Can you work these out from the model? Positions are in its coordinate system, mm. A direction names the side the tool comes from. Round coordinates to 2 decimals unless told otherwise and drop trailing zeros. Order: outer loops, then holes, each group sorted by start corner. A loop starts at its lowest first (then second) coordinate and runs counter-clockwise, first axis right, second up.
Q1. If we section it at C-C (y = 42): Please give me the cut outline in (x, z), plus the area to 3 significant figures.
Q2. If we section it at D-D (z = 2.1): Please give me the cut outline in (x, y).
Q3. If we section it at A-A (x = 8): Please give me the cut outline in (y, z).
Q4. If we section it at B-B (y = 8): Please give me the cut outline in (x, z).
Q5. Will these pins go through, and if not, where does the flat tip stop? P1, Ø1, axis at x = 25, z = 2.5, coming from the +Y side; P2, Ø2.5, axis at x = 42, y = 42, coming from the +Z side.
Q6. We'd pull the mould along Y, two halves only. Please class faces 1 (the face through (14, 25, 1)), 2 (the face through (30, 20, 0)), 3 (the face through (42, 44, 2)), 4 (the face through (0.86, 0.9, 1.52)): pulls with the +Y half, pulls with the -Y half, needs draft (parallel to the pull), parting line crosses it, or undercut.
Q7. If I drill on line 1 (X direction, y = 42, z = 1); line 2 (Y direction, x = 42, z = 2.2); line 3 (Y direction, x = 8, z = 1.2), over which ranges is the centre line in solid material (lowest first)?
Q8. For faces 5 (the face through (46.99, 2.85, 1.52)), 6 (the face through (25, 37, 1)), which set-ups out of +Z, -Z, +X, -X, +Y, -Y let a thin tool reach every point of the face, with its end or its side?
Autodesk Fusion 360 part; units mm, degrees
sketch "Sketch1" plane through (0, 0, 0) normal (0, 0, 1) x (1, 0, 0)
  line L0 (0, 0) -> (50, 0)
  line L1 (50, 0) -> (50, 50)
  line L2 (50, 50) -> (25, 50)
  line L3 (25, 50) -> (25, 25)
  line L4 (25, 25) -> (0, 25)
  line L5 (0, 25) -> (0, 0)
  line L6 (-25, 0) -> (-25, 55) construction
  dimension "d1" = 25
  dimension "d2" = 25
  dimension "d3" = 50
  dimension "d4" = 50
extrude "Extrude1" add sketch "Sketch1" along normal blind 3
ref_plane "WorkPlane1" through (-30, 0, 0) normal (1, 0, 0) x (0, 1, 0)
sketch "Sketch2" plane through (0, 0, 3) normal (0, 0, 1) x (-1, 0, 0)
  line L0 (0, -25) -> (0, 0)
  line L1 (0, 0) -> (-50, 0)
  line L2 (-50, 0) -> (-50, -50)
  line L3 (-50, -50) -> (-25, -50)
  line L4 (-25, -50) -> (-25, -25)
  line L5 (-25, -25) -> (0, -25)
  line L6 (-100, -100) -> (-70, -100)
  line L7 (-70, -100) -> (-70, -175)
  line L8 (-70, -175) -> (-100, -175)
  line L9 (-100, -175) -> (-100, -100)
  dimension "d10" = 30
  dimension "d11" = 75
fillet "Fillet1" radius 10 1 edges at (50, 0, 1.5)
fillet "Fillet2" radius 1 1 edges at (25, 25, 1.5)
fillet "Fillet3" radius 3 1 edges at (50, 50, 1.5)
fillet "Fillet4" radius 3 1 edges at (25, 50, 1.5)
fillet "Fillet5" radius 3 1 edges at (0, 25, 1.5)
fillet "Fillet6" radius 3 1 edges at (0, 0, 1.5)
sketch "Sketch5" plane through (0, 0, 3) normal (0, 0, 1) x (-1, 0, 0)
  arc A0 (0, -3) -> (-3, 0) centre (-3, -3) ccw
  line L0 (-3, 0) -> (-40, 0)
  arc A1 (-40, 0) -> (-50, -10) centre (-40, -10) ccw
  line L1 (-50, -10) -> (-50, -47)
  arc A2 (-50, -47) -> (-47, -50) centre (-47, -47) ccw
  line L2 (-47, -50) -> (-28, -50)
  arc A3 (-28, -50) -> (-25, -47) centre (-28, -47) ccw
  line L3 (-25, -47) -> (-25, -26)
  arc A4 (-24, -25) -> (-25, -26) centre (-24, -26) ccw
  line L4 (-24, -25) -> (-3, -25)
  arc A5 (-3, -25) -> (0, -22) centre (-3, -22) ccw
  line L5 (0, -22) -> (0, -3)
  circle A6 centre (-42, -8) radius 2
  circle A7 centre (-42, -42) radius 2
  circle A8 centre (-8, -8) radius 2
  dimension "d57" = 4
  dimension "d58" = 4
  dimension "d59" = 4
  dimension "d60" = 8
  dimension "d61" = 8
  dimension "d62" = 8
  dimension "d63" = 8
  dimension "d64" = 8
  dimension "d65" = 8
extrude "Extrude7" cut sketch "Sketch5" against normal blind 3 contours A6 | A7 | A8
Solution:
1. outline: (25, 0) - (40, 0) - (40, 3) - (25, 3) - close; (44, 0) - (50, 0) - (50, 3) - (44, 3) - close
1. area: 63.0 mm2
2. outline: (0, 3) arc R3 ccw to (3, 0) - (40, 0) arc R10 ccw to (50, 10) - (50, 47) arc R3 ccw to (47, 50) - (28, 50) arc R3 ccw to (25, 47) - (25, 26) arc R1 cw to (24, 25) - (3, 25) arc R3 ccw to (0, 22) - close; hole circle Ø4 at (8, 8); hole circle Ø4 at (42, 8); hole circle Ø4 at (42, 42)
3. outline: (0, 0) - (6, 0) - (6, 3) - (0, 3) - close; (10, 0) - (25, 0) - (25, 3) - (10, 3) - close
4. outline: (0, 0) - (6, 0) - (6, 3) - (0, 3) - close; (10, 0) - (40, 0) - (40, 3) - (10, 3) - close; (44, 0) - (49.8, 0) - (49.8, 3) - (44, 3) - close
5. P1: stops at y = 48.66
5. P2: passes through
6. face 1: pulls with the +Y half
6. face 2: needs draft
6. face 3: undercut
6. face 4: pulls with the -Y half
7. line 1: x = 25 to 40, 44 to 50
7. line 2: y = 0.2 to 6, 10 to 40, 44 to 50
7. line 3: y = 0 to 6, 10 to 25
8. face 5: +Z, -Z, +X, -Y
8. face 6: +Z, -Z, -X, +Y
